The model under review builds one solid part; all positions refer to its coordinate system, in mm. A direction names the side the tool comes from. Give positions to 0.01 mm unless a question says otherwise; leave off trailing zeros. Loops run counter-clockwise (first coordinate to the right, second up) from the corner with the lowest first, then second, coordinate; pieces in that order, holes last. Notation, with made-up numbers: M 78,62.25 L 95,62.25 A20 ccw 95,93.25 Z; hole C -22,71 d7. An arc over 180 degrees is marked long. Put each result on its own line as item: value. Start each with the question number.
from build123d import *

# Parameters (mm, degrees)
SKETCH_W     = 9.2
SKETCH_H     = 75
PAD_DEPTH    = 7.25
SKETCH001_W  = 4.2
SKETCH001_H  = 20.5
PAD001_DEPTH = 1.2
SKETCH002_R  = 0.35
PAD002_DEPTH = 3


with BuildPart() as part:
    # Sketch → Pad (new body)
    with BuildSketch(Plane.XY):
        Rectangle(SKETCH_W, SKETCH_H)
    extrude(amount=PAD_DEPTH)

    # Sketch001 (on Face2 of Pad) → Pad001 (join)
    with BuildSketch(Plane.YZ.offset(0.6)):
        with Locations((0, 11.5)):
            Rectangle(SKETCH001_W, SKETCH001_H)
    extrude(amount=-PAD001_DEPTH)

    # Sketch002 (on Face4 of Pad001) → Pad002 (join)
    with BuildSketch(Plane(origin=(0, 0, 0), x_dir=(1, 0, 0), z_dir=(0, 0, -1))):
        with Locations((-3.75, 35)):
            Circle(SKETCH002_R)
        with Locations((-1.25, 35)):
            Circle(SKETCH002_R)
        with Locations((1.25, 35)):
            Circle(SKETCH002_R)
        with Locations((3.75, 35)):
            Circle(SKETCH002_R)
        with Locations((3.75, -35)):
            Circle(SKETCH002_R)
        with Locations((-1.25, -35)):
            Circle(SKETCH002_R)
    extrude(amount=PAD002_DEPTH)


solid = part.part
(1) Insertion check: pin 1 (5 mm diameter, centred on x = 2.5, y = 13, fed in from -Z); pin 2 (1.3 mm diameter, centred on x = 0, z = 14, fed in from +Y); pin 3 (1.3 mm diameter, centred on y = -0.5, z = 11.5, fed in from +X). Each pin has a flat end and moves straight along its axis. Give the tip position at first contact, or say it passes through.
(2) We need section A-A, the plane y = -3. Write out the cut boundary in (x, z).
(3) We need section B-B, the plane z = 9. Write out the cut boundary in (x, y), plus the area to 3 significant figures.
(4) For faces 1 (the flat face through (-0.6, 0, 15)), 2 (the flat face through (0, -2.1, 14)), 3 (the flat face through (0, 2.1, 14)), list the 3-axis set-ups (+Z, -Z, +X, -X, +Y, -Y) from which the entire face can be reached by the end or side of a thin tool; tool diameter is ignored.
(5) To check wall thickness, follow L1, parallel to Z at x = -4, y = -16.5. State the ranges of the line that lie inside material, in increasing order. Write a range as [from, to].
Check sheet entries:
1. pin 1: stops at z = 0
1. pin 2: stops at y = 2.1
1. pin 3: stops at x = 0.6
2. outline: M -4.6,0 L 4.6,0 L 4.6,7.25 L -4.6,7.25 Z
3. outline: M -0.6,-2.1 L 0.6,-2.1 L 0.6,2.1 L -0.6,2.1 Z
3. area: 5.04 mm²
4. face 1: +Z, -X, +Y, -Y
4. face 2: +Z, +X, -X, -Y
4. face 3: +Z, +X, -X, +Y
5. L1: z = [0, 7.25]
